The model under review builds one solid part; all positions refer to its coordinate system, in mm. Face numbers are marked on the shaded views. Give positions to 0.01 mm unless a question says otherwise; leave off trailing zeros. Loops run counter-clockwise (first coordinate to the right, second up) from the corner with the lowest first, then second, coordinate; pieces in that order, holes last. Notation, with made-up numbers: M 18.25,-3.5 L 72.25,-3.5 A16 ccw 72.25,26.5 Z; hole C 23.25,66.5 d11. An arc over 180 degrees is marked long. One line per item, written item: value. Start each with the question number.
Q1. To check wall thickness, follow line 1 along Y through (x, z) = (0, 0.15); line 2 along Y through (x, z) = (0, 0.65); line 3 along X through (y, z) = (-0.5, 1.15). State the ranges of each line that lie inside material, in increasing order. Write a range as from..to.
Q2. We need section A-A on z = 0.8. Write out the cut boundary in (x, y).
Q3. Mouldability with a two-part tool opening along Y and no side actions: class the marked faces 1, 2, 3 and 4 as released by +Y, released by -Y, zero draft, split by the parting line, or undercut.
Q4. For pin 1 (5 mm diameter, centred on x = 1.5, y = 7, fed in from +Z); pin 2 (3 mm diameter, centred on x = 1, y = 1.5, fed in from +Z); pin 3 (1 mm diameter, centred on y = 3.5, z = 2, fed in from -X), all flat-tipped, find the tip position at first contact; note any pin that passes through.
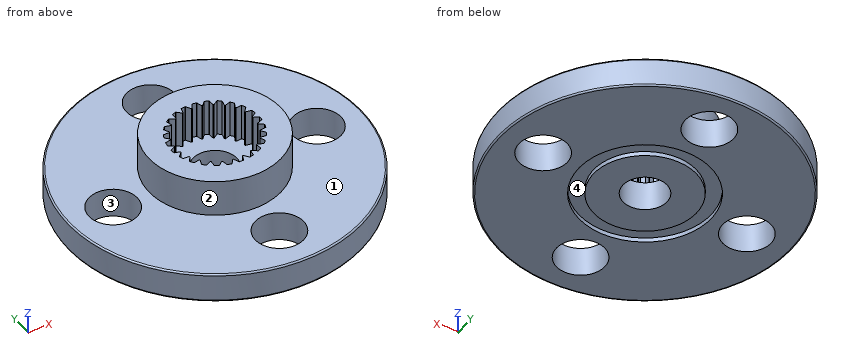
```python
from build123d import *

# Parameters (mm, degrees)
SKETCH3_R           = 10
SKETCH3_R_2         = 1.5
BOSS_EXTRUDE2_DEPTH = 2
FILLET1_R           = 0.1
SKETCH5_R           = 4.5
SKETCH5_R_2         = 3
BOSS_EXTRUDE3_DEPTH = 2.5
SKETCH6_R           = 4.5
SKETCH6_R_2         = 3.5
CUT_EXTRUDE3_DEPTH  = 0.3
BOSS_EXTRUDE1_DEPTH = 4.5
CIRPATTERN6_COUNT   = 25
CUT_EXTRUDE4_REACH  = 16.361
SKETCH8_R           = 1.65


with BuildPart() as part:
    # Sketch3 → Boss-Extrude2 (new body)
    with BuildSketch(Plane.XY):
        Circle(SKETCH3_R)
        Circle(SKETCH3_R_2, mode=Mode.SUBTRACT)
    extrude(amount=BOSS_EXTRUDE2_DEPTH)

    # Fillet1
    fillet1_edges = [part.edges().sort_by_distance(p)[0] for p in [
        (-10, 0, 0),
        (-10, 0, 2),
    ]]
    fillet(fillet1_edges, radius=FILLET1_R)

    # Sketch5 → Boss-Extrude3 (add)
    with BuildSketch(Plane.XY.offset(2)):
        Circle(SKETCH5_R)
        Circle(SKETCH5_R_2, mode=Mode.SUBTRACT)
    extrude(amount=BOSS_EXTRUDE3_DEPTH)

    # Sketch6 → Cut-Extrude3 (cut)
    with BuildSketch(Plane(origin=(0, 0, 0), x_dir=(-1, 0, 0), z_dir=(0, 0, -1))):
        with Locations(Location((0, 0, 0), (0, 0, 180))):
            Circle(SKETCH6_R)
        Circle(SKETCH6_R_2, mode=Mode.SUBTRACT)
    extrude(amount=-CUT_EXTRUDE3_DEPTH, mode=Mode.SUBTRACT)

    # Sketch2 → Boss-Extrude1 (add)
    with BuildSketch(Plane.XY):
        Polygon((-0.224920346, -2.97556486), (-0.224920346, -3.054661592), (-0.671931157, -3.032807749), (-0.671931157, -2.923783255), (-0.433398187, -2.602688219), (-0.383730319, -2.608441731), align=None)
    boss_extrude1 = extrude(amount=BOSS_EXTRUDE1_DEPTH)

    # CirPattern6: Boss-Extrude1 ×25 about axis
    cirpattern6_axis = Axis((0, 0, 0), (0, 0, 1))
    for i in range(1, CIRPATTERN6_COUNT):
        add(boss_extrude1.rotate(cirpattern6_axis, i * 360 / CIRPATTERN6_COUNT))

    # Sketch8 → Cut-Extrude4 (cut, up to next)
    with BuildSketch(Plane.XY.offset(2), mode=Mode.PRIVATE) as cut_extrude4_sk1:
        with Locations((0, 7)):
            Circle(SKETCH8_R)
    cut_extrude4_tool1 = extrude(cut_extrude4_sk1.sketch, amount=-CUT_EXTRUDE4_REACH, mode=Mode.PRIVATE) & part.part
    # Sketch8 → Cut-Extrude4 (cut, up to next)
    with BuildSketch(Plane.XY.offset(2), mode=Mode.PRIVATE) as cut_extrude4_sk2:
        with Locations((0, -7)):
            Circle(SKETCH8_R)
    cut_extrude4_tool2 = extrude(cut_extrude4_sk2.sketch, amount=-CUT_EXTRUDE4_REACH, mode=Mode.PRIVATE) & part.part
    # Sketch8 → Cut-Extrude4 (cut, up to next)
    with BuildSketch(Plane.XY.offset(2), mode=Mode.PRIVATE) as cut_extrude4_sk3:
        with Locations((7, 0)):
            Circle(SKETCH8_R)
    cut_extrude4_tool3 = extrude(cut_extrude4_sk3.sketch, amount=-CUT_EXTRUDE4_REACH, mode=Mode.PRIVATE) & part.part
    # Sketch8 → Cut-Extrude4 (cut, up to next)
    with BuildSketch(Plane.XY.offset(2), mode=Mode.PRIVATE) as cut_extrude4_sk4:
        with Locations((-7, 0)):
            Circle(SKETCH8_R)
    cut_extrude4_tool4 = extrude(cut_extrude4_sk4.sketch, amount=-CUT_EXTRUDE4_REACH, mode=Mode.PRIVATE) & part.part
    add(cut_extrude4_tool1.solids().sort_by_distance((0, 7, 2))[0], mode=Mode.SUBTRACT)
    add(cut_extrude4_tool2.solids().sort_by_distance((0, -7, 2))[0], mode=Mode.SUBTRACT)
    add(cut_extrude4_tool3.solids().sort_by_distance((7, 0, 2))[0], mode=Mode.SUBTRACT)
    add(cut_extrude4_tool4.solids().sort_by_distance((-7, 0, 2))[0], mode=Mode.SUBTRACT)


solid = part.part
```
Solved:
1. line 1: -10..-8.65, -5.35..-4.5, -3.5..-1.5, 1.5..3.5, 4.5..5.35, 8.65..10
1. line 2: -10..-8.65, -5.35..-1.5, 1.5..5.35, 8.65..10
1. line 3: -9.99..-8.57, -5.43..-1.41, 1.41..5.43, 8.57..9.99
2. outline: C 0,0 d20; hole C -7,0 d3.3; hole C 0,-7 d3.3; hole C 0,7 d3.3; hole C 0,0 d3; hole C 7,0 d3.3
3. face 1: zero draft
3. face 2: split by the parting line
3. face 3: undercut
3. face 4: undercut
4. pin 1: z = 2
4. pin 2: z = 4.5
4. pin 3: x = -9.54
